Geometry: final body of the model. Coordinates: model frame, mm. Face numbers are marked on the shaded views. A direction names the side the tool comes from. Coordinates: 2 decimals unless noted, no trailing zeros. Order: outer loops, then holes, each group sorted by start corner. A loop starts at its lowest first (then second) coordinate and runs counter-clockwise, first axis right, second up. Notation, with made-up numbers: (24, -10.75) -> (76, -10.75) arc R29 cw to (76, 15.25) -> close; hole circle Ø3 at (-22.5, -32.5). An arc over 180 degrees is marked (long way). Use one line per item in the form item = value.
```python
from build123d import *

# Parameters (mm, degrees)
BOSS_EXTRU_1_DEPTH      = 15
ESQUISSE3_R             = 5
ESQUISSE3_W             = 60
ESQUISSE3_H             = 15
ESQUISSE3_W_2           = 10
ESQUISSE3_H_2           = 50
ESQUISSE3_W_3           = 25
ESQUISSE3_H_3           = 10
ENL_V_MAT_EXTRU_1_DEPTH = 15


with BuildPart() as part:
    # Esquisse2 → Boss.-Extru.1 (new body)
    with BuildSketch(Plane.XY):
        with BuildLine():
            Line((-50, 0), (50, 0))
            Line((50, 0), (50, 15))
            Line((50, 15), (29.792740578, 50))
            Line((29.792740578, 50), (29.792740578, 70))
            Line((29.792740578, 70), (19.792740578, 70))
            Line((19.792740578, 70), (19.792740578, 85))
            Line((19.792740578, 85), (29.792740578, 85))
            Line((29.792740578, 85), (29.792740578, 90))
            ThreePointArc((29.792740578, 90), (26.86380839, 97.071067812), (19.792740578, 100))
            Line((19.792740578, 100), (-19.792740578, 100))
            ThreePointArc((-19.792740578, 100), (-26.86380839, 97.071067812), (-29.792740578, 90))
            Line((-29.792740578, 90), (-29.792740578, 85))
            Line((-29.792740578, 85), (-19.792740578, 85))
            Line((-19.792740578, 85), (-19.792740578, 70))
            Line((-19.792740578, 70), (-29.792740578, 70))
            Line((-29.792740578, 70), (-29.792740578, 50))
            Line((-29.792740578, 50), (-50, 15))
            Line((-50, 15), (-50, 0))
        make_face()
    extrude(amount=BOSS_EXTRU_1_DEPTH)

    # Esquisse3 → Enlèv. mat.-Extru.1 (cut)
    with BuildSketch(Plane.XY.offset(15)):
        with Locations((0, 77.5)):
            Circle(ESQUISSE3_R)
        with Locations((0, 7.5)):
            Rectangle(ESQUISSE3_W, ESQUISSE3_H)
        with Locations((0, 25)):
            Rectangle(ESQUISSE3_W_2, ESQUISSE3_H_2)
        with Locations((0, 36.515847226)):
            Rectangle(ESQUISSE3_W_3, ESQUISSE3_H_3)
    extrude(amount=-ENL_V_MAT_EXTRU_1_DEPTH, mode=Mode.SUBTRACT)


solid = part.part
```
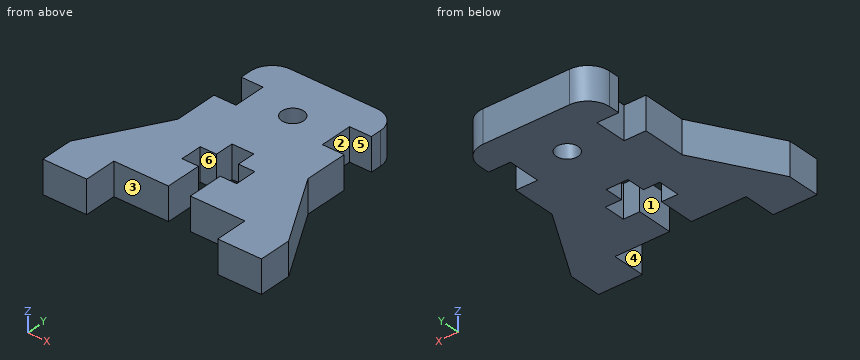
1) Access query for the marked faces 4, 5 and 6. Directions: +Z, -Z, +X, -X, +Y, -Y. A direction counts if a zero-diameter tool reaches every point of the face in a straight line with its end or side. Return the directions, or none.
Results found:
face_4 = +Z, -Z, -Y
face_5 = +Z, -Z, +X
face_6 = +Z, -Z
2) Section C-C, the plane x = 18. Output: boundary loops of the cut face in (y, z), and give its area (4 significant figures).
Results found:
outline = (15, 0) -> (100, 0) -> (100, 15) -> (15, 15) -> close
area = 1,275 mm2
3) Pull-direction query (Y, two-part tool) for the marked faces 1, 2 and 3; classes: released by +Y, released by -Y, zero draft, split by the parting line, or undercut.
Results found:
face_1 = zero draft
face_2 = undercut
face_3 = released by -Y
4) Material intervals for probe 1 along Y at (x, z) = (10.5, 14); probe 2 along Y at (x, z) = (0, 5); probe 3 along X at (y, z) = (10, 10.5), sorted ascending. Write a range as from..to.
Results found:
probe_1 = 15..31.52, 41.52..100
probe_2 = 50..72.5, 82.5..100
probe_3 = -50..-30, 30..50
5) Section A-A, the plane x = 0. Output: boundary loops of the cut face in (y, z), and give its area (3 significant figures).
Results found:
outline = (50, 0) -> (72.5, 0) -> (72.5, 15) -> (50, 15) -> close; (82.5, 0) -> (100, 0) -> (100, 15) -> (82.5, 15) -> close
area = 600 mm2
6) Section B-B, the plane y = 77.5. Output: boundary loops of the cut face in (x, z), and give its area (3 significant figures).
Results found:
outline = (-19.79, 0) -> (-5, 0) -> (-5, 15) -> (-19.79, 15) -> close; (5, 0) -> (19.79, 0) -> (19.79, 15) -> (5, 15) -> close
area = 444 mm2
7) Section D-D, the plane x = -34. Output: boundary loops of the cut face in (y, z), and give its area (3 significant figures).
Results found:
outline = (0, 0) -> (42.71, 0) -> (42.71, 15) -> (0, 15) -> close
area = 641 mm2
8) Contact query for flat-ended pins moving along their axis: P1, Ø1.5, axis at y = 88, z = 7.5, coming from the -X side; P2, Ø1.5, axis at y = 63, z = 13, coming from the +X side; P3, Ø3, axis at x = -26.5, z = 9.5, coming from the +Y side. Output: stop coordinate, or through.
Results found:
P1 = -29.79
P2 = 29.79
P3 = 98.54
